Source: three-view drawing plus pictorial views. Frame: mm from the lowest corner of the part. A direction names the side the tool comes from. Round coordinates to 2 decimals unless told otherwise and drop trailing zeros. Loops run counter-clockwise (first coordinate to the right, second up) from the corner with the lowest first, then second, coordinate; pieces in that order, holes last. Notation, with made-up numbers: M 31,36.5 L 75,36.5 A12 cw 75,49.5 Z; hole C -25.75,77.5 d10. An arc over 180 degrees is marked long. Answer as a JSON object with one key per item and string values.
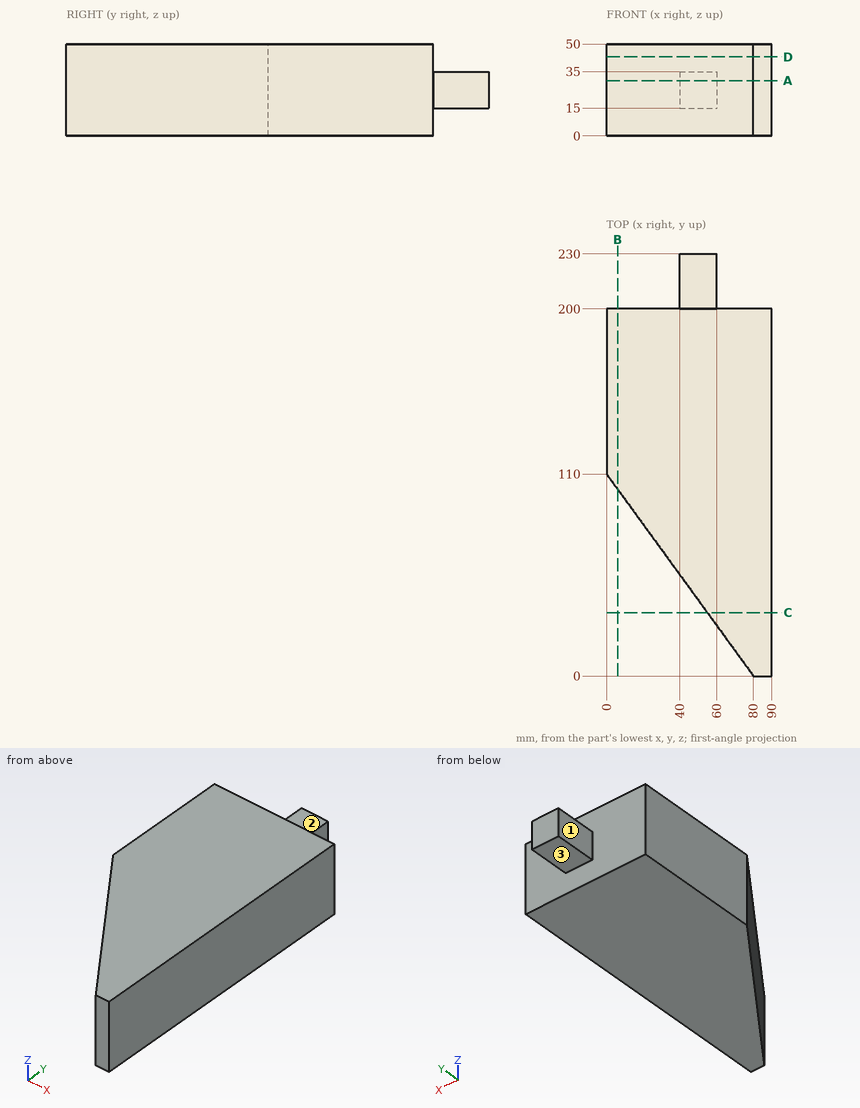
1) Set-up query: the marked faces 1, 2 and 3. Return all of +Z, -Z, +X, -X, +Y, -Y with unobstructed straight access to the full face (end or side cutting, diameter ignored); none if empty.
Geometry results:
{"face 1": "+Z, -Z, -X, +Y", "face 2": "+Z, +X, -X, +Y", "face 3": "-Z, +X, -X, +Y"}
2) First-contact query: pin 1 (16 mm diameter, centred on y = 218, z = 21.5, fed in from -X); pin 2 (12 mm diameter, centred on x = 63, z = 22.5, fed in from -Y) (3 decimals); pin 3 (1.5 mm diameter, centred on x = 23, z = 37, fed in from -Y). Flat tips, straight axial feed; report the tip coordinate or a pass-through.
Geometry results:
{"pin 1": "x = 40", "pin 2": "y = 15.125", "pin 3": "y = 77.34"}
3) Line query: probe 1 along Y at (x, z) = (70.5, 48); probe 2 along Y at (x, z) = (23, 16) (3 decimals); probe 3 along X at (y, z) = (57.5, 18). Output: solid intervals per line, ascending.
Geometry results:
{"probe 1": "13.06 to 200", "probe 2": "78.375 to 200", "probe 3": "38.18 to 90"}
4) Cut plane C-C on y = 34.5. Return the cut outline in (x, z).
Geometry results:
{"outline": "M 54.91,0 L 90,0 L 90,50 L 54.91,50 Z"}
5) Cut plane B-B on x = 6. Return the cut outline in (y, z).
Geometry results:
{"outline": "M 101.75,0 L 200,0 L 200,50 L 101.75,50 Z"}
6) Cut plane D-D on z = 43. Return the cut outline in (x, y), and give its area (3 significant figures).
Geometry results:
{"outline": "M 0,110 L 80,0 L 90,0 L 90,200 L 0,200 Z", "area": "13,600 mm2"}
7) Cut plane A-A on z = 30. Return the cut outline in (x, y).
Geometry results:
{"outline": "M 0,110 L 80,0 L 90,0 L 90,200 L 60,200 L 60,230 L 40,230 L 40,200 L 0,200 Z"}
